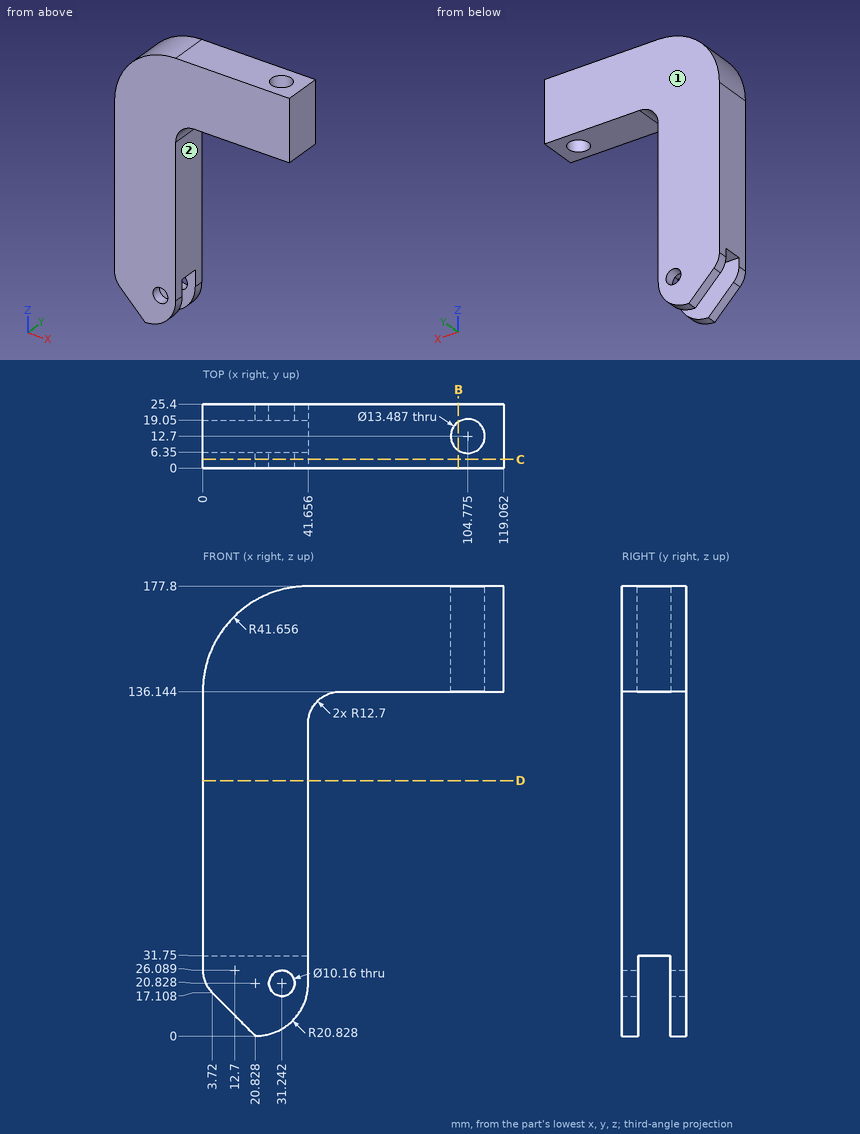
Could you check a few things on this drawing? It's one solid part, dimensions in mm from its lowest x, y, z. A direction names the side the tool comes from. Give positions to 0.01 mm unless a question says otherwise; leave off trailing zeros. Order: outer loops, then holes, each group sorted by start corner. A loop starts at its lowest first (then second) coordinate and runs counter-clockwise, first axis right, second up. Notation, with made-up numbers: M 31.25,80 L 64.25,80 A24 cw 64.25,100 Z; hole C 5.5,-6 d6. An arc over 180 degrees is marked long. Use one line per item in the form item = value. Start each with the question number.
Item 1: If we section it at C-C (y = 3.5): Write out the boundary of the cut face in (x, z) (1 decimal), then the cut area to 3 significant figures.
Item 2: If I drill on line 1 along X through (y, z) = (14.5, 87) (1 decimal); line 2 along Z through (x, y) = (87, 8.5) (1 decimal); line 3 along X through (y, z) = (8.75, 154), over which ranges is the centre line in solid material (lowest first)?
Item 3: For the marked faces 1 and 2, which set-ups out of +Z, -Z, +X, -X, +Y, -Y let a thin tool reach every point of the face, with its end or its side?
Item 4: If we section it at D-D (z = 101): Write out the boundary of the cut face in (x, y) (1 decimal), then the cut area to 3 significant figures.
Item 5: Will these pins go through, and if not, where does the flat tip stop? pin 1 Ø6 at (x, y) = (21.5, 16.5) entering from +Z; pin 2 Ø4 at (x, y) = (22, 13) entering from -Z; pin 3 Ø12.5 at (x, y) = (80, 11) entering from -Z.
Item 6: If we section it at B-B (x = 101): Write out the boundary of the cut face in (y, z) (1 decimal).
Outcome:
q1.outline = M 0,26.1 A12.7 ccw 3.7,17.1 L 20.8,0 A20.8 ccw 41.7,20.8 L 41.7,123.4 A12.7 cw 54.4,136.1 L 119.1,136.1 L 119.1,177.8 L 41.7,177.8 A41.7 ccw 0,136.1 Z; hole C 31.2,20.8 d10.2
q1.area = 9,900 mm2
q2.line_1 = 0 to 41.7
q2.line_2 = 136.1 to 177.8
q2.line_3 = 4.02 to 99.31, 110.24 to 119.06
q3.face_1 = +Z, -Z, +X, -X, +Y
q3.face_2 = -Z, +X, +Y, -Y
q4.outline = M 0,0 L 41.7,0 L 41.7,25.4 L 0,25.4 Z
q4.area = 1,060 mm2
q5.pin_1 = 174.1
q5.pin_2 = 31.75
q5.pin_3 = 136.14
q6.outline = M 0,136.1 L 7.1,136.1 L 7.1,177.8 L 0,177.8 Z; M 18.3,136.1 L 25.4,136.1 L 25.4,177.8 L 18.3,177.8 Z
